```python
from build123d import *

# Parameters (mm, degrees)
SKETCH_1_W          = 42
SKETCH_1_H          = 42
SKETCH_1_R          = 1.6
SKETCH_1_R_2        = 12
EXTRUDE_1_DEPTH     = 3
SKETCH_2_W          = 16
SKETCH_2_H          = 36
EXTRUDE_2_DEPTH     = 10
SKETCH_3_R          = 4.4
CUT_EXTRUDE_1_DEPTH = 6
EXTRUDE_3_DEPTH     = 65
SKETCH_5_W          = 6.2
SKETCH_5_H          = 20
CUT_EXTRUDE_2_DEPTH = 50
CUT_EXTRUDE_3_REACH = 84.644
SKETCH_6_W          = 6.2
SKETCH_6_H          = 20
SKETCH_7_W          = 16
SKETCH_7_H          = 0.6
CUT_EXTRUDE_4_DEPTH = 33


with BuildPart() as part:
    # 草图1 → 凸台-拉伸1 (new body)
    with BuildSketch(Plane(origin=(0, 0, 0), x_dir=(1, 0, 0), z_dir=(0, 1, 0))):
        Rectangle(SKETCH_1_W, SKETCH_1_H)
        with Locations(Location((15.5, 15.5, 0), (0, 0, 270))):
            Circle(SKETCH_1_R, mode=Mode.SUBTRACT)
        with Locations(Location((15.5, -15.5, 0), (0, 0, 270))):
            Circle(SKETCH_1_R, mode=Mode.SUBTRACT)
        with Locations(Location((-15.5, -15.5, 0), (0, 0, 270))):
            Circle(SKETCH_1_R, mode=Mode.SUBTRACT)
        with Locations(Location((-15.5, 15.5, 0), (0, 0, 270))):
            Circle(SKETCH_1_R, mode=Mode.SUBTRACT)
        with Locations(Location((0, 0, 0), (0, 0, 270))):
            Circle(SKETCH_1_R_2, mode=Mode.SUBTRACT)
    extrude(amount=EXTRUDE_1_DEPTH)

    # 草图2 → 凸台-拉伸2 (add)
    with BuildSketch(Plane.XY.offset(21)):
        with Locations((0, -15)):
            Rectangle(SKETCH_2_W, SKETCH_2_H)
    extrude(amount=EXTRUDE_2_DEPTH)

    # 草图3 → 切除-拉伸1 (cut)
    with BuildSketch(Plane.XY.offset(31)):
        with Locations((0, -9)):
            Circle(SKETCH_3_R)
    extrude(amount=-CUT_EXTRUDE_1_DEPTH, mode=Mode.SUBTRACT)

    # 草图4 → 凸台-拉伸3 (add)
    with BuildSketch(Plane(origin=(0, 3, 0), x_dir=(1, 0, 0), z_dir=(0, 1, 0))):
        Polygon((1, 21), (21, 21), (21, 1), (24, 1), (24, 24), (1, 24), align=None)
    extrude(amount=-EXTRUDE_3_DEPTH)

    # 草图5 → 切除-拉伸2 (cut)
    with BuildSketch(Plane(origin=(0, 0, -24), x_dir=(-1, 0, 0), z_dir=(0, 0, -1))):
        with Locations((-11, -52)):
            Rectangle(SKETCH_5_W, SKETCH_5_H)
    extrude(amount=-CUT_EXTRUDE_2_DEPTH, mode=Mode.SUBTRACT)

    # 草图6 → 切除-拉伸3 (cut, up to next)
    with BuildSketch(Plane(origin=(24, 0, 0), x_dir=(0, 0, -1), z_dir=(1, 0, 0)), mode=Mode.PRIVATE) as cut_extrude_3_sk1:
        with Locations((11, -52)):
            Rectangle(SKETCH_6_W, SKETCH_6_H)
    cut_extrude_3_tool1 = extrude(cut_extrude_3_sk1.sketch, amount=-CUT_EXTRUDE_3_REACH, mode=Mode.PRIVATE) & part.part
    add(cut_extrude_3_tool1.solids().sort_by_distance((24, -52, -11))[0], mode=Mode.SUBTRACT)

    # 草图7 → 切除-拉伸4 (cut)
    with BuildSketch(Plane.XZ.offset(33)):
        with Locations((0, 21.3)):
            Rectangle(SKETCH_7_W, SKETCH_7_H)
    extrude(amount=-CUT_EXTRUDE_4_DEPTH, mode=Mode.SUBTRACT)


with BuildPart() as body_2:
    # 镜向3: mirrored copy
    add(part.part.mirror(Plane.ZY.offset(31)))


solid = body_2.part
```
Work out the finished part from the listing and answer in its coordinate system (mm). A direction names the side the tool comes from. Round coordinates to 2 decimals unless told otherwise and drop trailing zeros. Loops run counter-clockwise (first coordinate to the right, second up) from the corner with the lowest first, then second, coordinate; pieces in that order, holes last. Notation, with made-up numbers: M 5.5,65.25 L 15.5,65.25 A27 cw 15.5,84.25 Z; hole C 41.25,78 d8. An arc over 180 degrees is marked long. Use CSV: the item, a comma, the result in double quotes.
Q1. Section B-B, the plane z = 15.5 is taken. Determine the outline of the cut face in (x, y).
Determined:
outline,"M -83,0 L -79.1,0 L -79.1,3 L -83,3 Z; M -75.9,0 L -48.1,0 L -48.1,3 L -75.9,3 Z; M -44.9,0 L -41,0 L -41,3 L -44.9,3 Z"
Q2. Section C-C, the plane x = -68 is taken. Determine the outline of the cut face in (y, z).
Determined:
outline,"M -62,-24 L 3,-24 L 3,-10.39 L 0,-10.39 L 0,-21 L -62,-21 Z; M -33,21.6 L 0,21.6 L 0,10.39 L 3,10.39 L 3,31 L -33,31 Z"
Q3. A tool of negligible diameter and unlimited length cuts with its end or side. For faces 4 (the flat face through (-62, -9, 25)), 5 (the flat face through (-73, -31, -21)), 6 (the flat face through (-54, -15, 26)), from which of +Z, -Z, +X, -X, +Y, -Y can it reach the whole face along a straight path? Write none if from no direction.
Determined:
face 4,"+Z"
face 5,"+X, -Y"
face 6,"+Z, +X, +Y, -Y"
Q4. Section D-D, the plane y = -27 is taken. Determine the outline of the cut face in (x, z), then the cut area to 3 significant figures.
Determined:
outline,"M -86,-24 L -63,-24 L -63,-21 L -83,-21 L -83,-1 L -86,-1 Z; M -70,21.6 L -54,21.6 L -54,31 L -70,31 Z"
area,"279 mm2"
Q5. The mould has two halves that part along X. Classify faces 1 (the flat face through (-63, -29, -23)), 2 (the cylindrical face through (-45.53, 1.48, -16.77)), 3 (the flat face through (-82.1, -62, -21.3)): pulls with the +X half, pulls with the -X half, needs draft (parallel to the pull), parting line crosses it, or undercut.
Determined:
face 1,"pulls with the +X half"
face 2,"undercut"
face 3,"needs draft"
Q6. Section A-A, the plane y = -55.5 is taken. Determine the outline of the cut face in (x, z).
Determined:
outline,"M -86,-24 L -76.1,-24 L -76.1,-21 L -83,-21 L -83,-14.1 L -86,-14.1 Z; M -86,-7.9 L -83,-7.9 L -83,-1 L -86,-1 Z; M -69.9,-24 L -63,-24 L -63,-21 L -69.9,-21 Z"
Q7. Consider L1, parallel to Z at x = -46.5, y = 1.9; L2, parallel to X at y = 1.55, z = -15.5; L3, parallel to X at y = 2, z = 0. Determine where each line is inside the solid, lowest interval first.
Determined:
L1,"-21 to -17.1, -13.9 to 13.9, 17.1 to 21"
L2,"-86 to -79.1, -75.9 to -48.1, -44.9 to -41"
L3,"-83 to -74, -50 to -41"
Q8. Each of these flat-tipped pins is pushed along its axis until it touches: pin 1 (0.9 mm diameter, centred on y = -49, z = -23, fed in from +X); pin 2 (2.5 mm diameter, centred on x = -50, y = 2, fed in from +Z); pin 3 (2.5 mm diameter, centred on x = -72.5, z = -23, fed in from -Y); pin 4 (5 mm diameter, centred on x = -59, y = -48.5, fed in from -Z). Where does it stop, or does it pass through?
Determined:
pin 1,"x = -63"
pin 2,"z = 21"
pin 3,"y = -42"
pin 4,"through"
